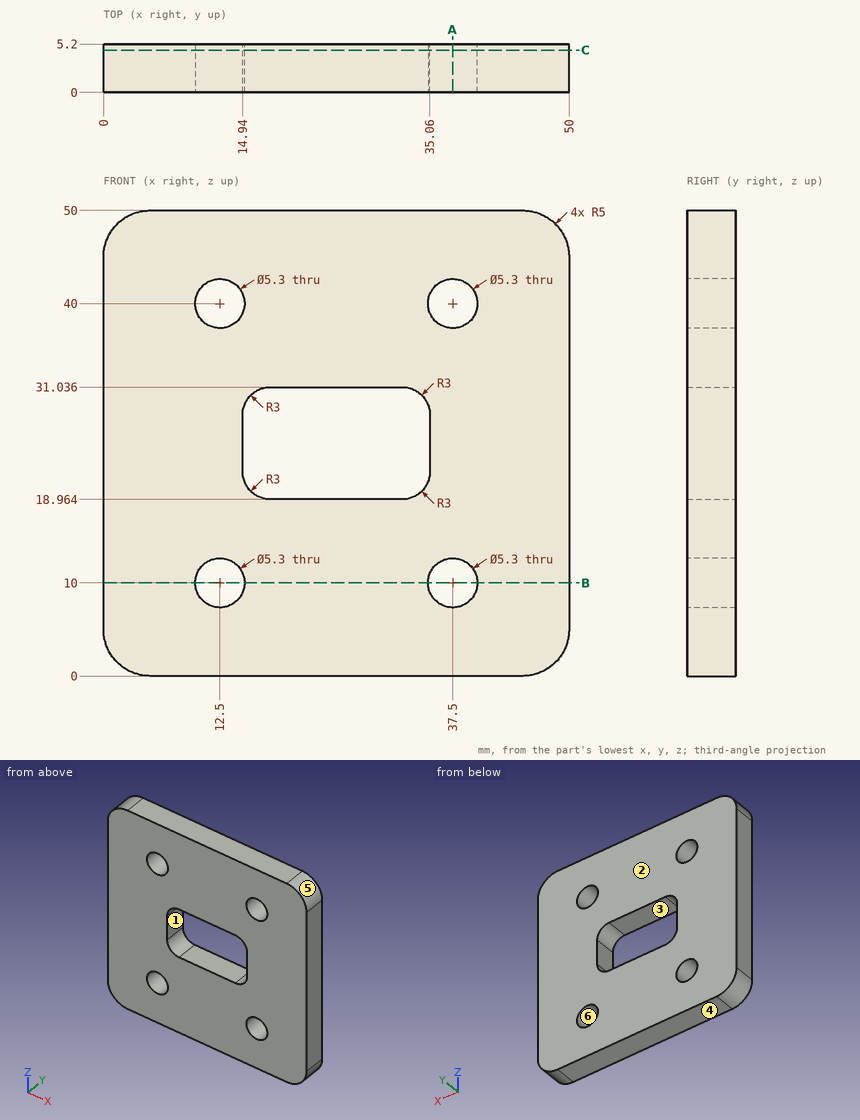
Here's the drawing with two shaded views (mm, measured from the low corner). I have some questions. A direction names the side the tool comes from. Round coordinates to 2 decimals unless told otherwise and drop trailing zeros. Loops run counter-clockwise (first coordinate to the right, second up) from the corner with the lowest first, then second, coordinate; pieces in that order, holes last. Notation, with made-up numbers: (89, 50) - (122, 50) arc R23 ccw to (122, 81) - close; hole circle Ø10 at (-24.5, 12.25). An arc over 180 degrees is marked (long way). Use CSV: the item, a comma, the result in double quotes.
Item 1: If we section it at B-B on z = 10: List the corners of the cut face in (x, y) for me.
Here are the results:
outline,"(0, 0) - (9.85, 0) - (9.85, 5.2) - (0, 5.2) - close; (15.15, 0) - (34.85, 0) - (34.85, 5.2) - (15.15, 5.2) - close; (40.15, 0) - (50, 0) - (50, 5.2) - (40.15, 5.2) - close"
Item 2: I need wall thicknesses on L1, parallel to X at y = 1.35, z = 10; L2, parallel to Z at x = 12.5, y = 2.2; L3, parallel to Z at x = 10.5, y = 4.65. Which ranges of each line are inside material? Lowest first, please. Write a range as [from, to].
Here are the results:
L1,"x = [0, 9.85], [15.15, 34.85], [40.15, 50]"
L2,"z = [0, 7.35], [12.65, 37.35], [42.65, 50]"
L3,"z = [0, 8.26], [11.74, 38.26], [41.74, 50]"
Item 3: For the marked faces 1 and 2, which set-ups out of +Z, -Z, +X, -X, +Y, -Y let a thin tool reach every point of the face, with its end or its side?
Here are the results:
face 1,"+Y, -Y"
face 2,"+Z, -Z, +X, -X, +Y"
Item 4: If we mould it in two halves opening along X, with no side actions, what happens to the marked faces 3, 4, 5 and 6? For each: pulls with the +X half, pulls with the -X half, needs draft (parallel to the pull), parting line crosses it, or undercut.
Here are the results:
face 3,"undercut"
face 4,"needs draft"
face 5,"pulls with the +X half"
face 6,"undercut"
Item 5: If we section it at A-A on x = 37.5: List the corners of the cut face in (y, z) for me.
Here are the results:
outline,"(0, 0) - (5.2, 0) - (5.2, 7.35) - (0, 7.35) - close; (0, 12.65) - (5.2, 12.65) - (5.2, 37.35) - (0, 37.35) - close; (0, 42.65) - (5.2, 42.65) - (5.2, 50) - (0, 50) - close"
Item 6: If we section it at C-C on y = 4.55: List the corners of the cut face in (x, z) for me, then the cut area to 4 significant figures.
Here are the results:
outline,"(0, 5) arc R5 ccw to (5, 0) - (45, 0) arc R5 ccw to (50, 5) - (50, 45) arc R5 ccw to (45, 50) - (5, 50) arc R5 ccw to (0, 45) - close; hole circle Ø5.3 at (12.5, 10); hole circle Ø5.3 at (12.5, 40); hole (14.94, 21.96) arc R3 ccw to (17.94, 18.96) - (32.06, 18.96) arc R3 ccw to (35.06, 21.96) - (35.06, 28.04) arc R3 ccw to (32.06, 31.04) - (17.94, 31.04) arc R3 ccw to (14.94, 28.04) - close; hole circle Ø5.3 at (37.5, 10); hole circle Ø5.3 at (37.5, 40)"
area,"2,155 mm²"
